For this review, take the finished solid that the model builds, in its own axes (mm). Round coordinates to 2 decimals unless told otherwise and drop trailing zeros. Write each loop counter-clockwise with the first axis right and the second up, starting at its lowest first coordinate (ties: lowest second). Pieces come first, ordered by that corner, then holes. Notation, with made-up numbers: (8, 59) -> (35, 59) arc R28 ccw to (35, 88) -> close; hole circle Ø1 at (-20, 27). An arc over 180 degrees is marked (long way). Answer as CSV lines item,"result". Start each with the question number.
Item 1: Take a section at B-B on z = 657.5. Give the boundary of the cut face in (x, y), then the cut area to 3 significant figures.
Item 2: Take a section at A-A on y = -20. Give the boundary of the cut face in (x, z), then the cut area to 3 significant figures.
Item 3: Wall thickness on probe 1 along X at (y, z) = (-5, 666); probe 2 along X at (y, z) = (-4, 436.5); probe 3 along Y at (x, z) = (17.5, 52.5): over which ranges is each line inside the solid? List them lowest first. Write a range as from..to.
Item 4: For pin 1 Ø10 at (x, y) = (13.5, -9.5) entering from -Z (3 decimals), flat-tipped, find the tip position at first contact; note if it passes through.
Item 5: Mouldability with a two-part tool opening along X and no side actions: class faces 1 (the flat face through (32.5, -15, 493)), 2 (the flat face through (16.1, -1.6, 0)), 3 (the flat face through (30.5, -16, 493)), 4 (the flat face through (1.5, -16, 493)) as +X half, -X half, draft (parallel to the pull), parting line (faces both ways), or undercut.
```python
from build123d import *

# Parameters (mm, degrees)
EXTRUDE_1_DEPTH = 1000


with BuildPart() as part:
    # 草图1 → 凸台-拉伸1 (new body)
    with BuildSketch(Plane.XY):
        with BuildLine():
            Line((10.5, -30), (0, -30))
            ThreePointArc((0, -30), (-0.353553391, -29.853553391), (-0.5, -29.5))
            Line((-0.5, -29.5), (-0.5, -0.5))
            ThreePointArc((-0.5, -0.5), (-0.353553391, -0.146446609), (0, 0))
            Line((0, 0), (32, 0))
            ThreePointArc((32, 0), (32.353553391, -0.146446609), (32.5, -0.5))
            Line((32.5, -0.5), (32.5, -29.5))
            ThreePointArc((32.5, -29.5), (32.353553391, -29.853553391), (32, -30))
            Line((32, -30), (21.5, -30))
            Line((21.5, -30), (21.5, -27))
            ThreePointArc((21.5, -27), (25.038664483, -28.385121551), (28.838528773, -28.426827781))
            ThreePointArc((28.838528773, -28.426827781), (30.029224893, -27.744667111), (30.5, -26.455686418))
            Line((30.5, -26.455686418), (30.5, -5))
            ThreePointArc((30.5, -5), (29.621320344, -2.878679656), (27.5, -2))
            Line((27.5, -2), (21.562207583, -2))
            Line((21.562207583, -2), (21.175427925, -2.706444665))
            ThreePointArc((21.175427925, -2.706444665), (21, -2.810397577), (20.824572075, -2.706444665))
            Line((20.824572075, -2.706444665), (20.437792417, -2))
            Line((20.437792417, -2), (11.562207583, -2))
            Line((11.562207583, -2), (11.175427925, -2.706444665))
            ThreePointArc((11.175427925, -2.706444665), (11, -2.810397577), (10.824572075, -2.706444665))
            Line((10.824572075, -2.706444665), (10.437792417, -2))
            Line((10.437792417, -2), (4.5, -2))
            ThreePointArc((4.5, -2), (2.378679656, -2.878679656), (1.5, -5))
            Line((1.5, -5), (1.5, -26.455686418))
            ThreePointArc((1.5, -26.455686418), (1.970775107, -27.744667111), (3.161471227, -28.426827781))
            ThreePointArc((3.161471227, -28.426827781), (6.961335517, -28.385121551), (10.5, -27))
            Line((10.5, -27), (10.5, -30))
        make_face()
    extrude(amount=EXTRUDE_1_DEPTH)


solid = part.part
```
Output values:
1,outline,"(-0.5, -29.5) arc R0.5 ccw to (0, -30) -> (10.5, -30) -> (10.5, -27) arc R10.55 cw to (3.16, -28.43) arc R2 cw to (1.5, -26.46) -> (1.5, -5) arc R3 cw to (4.5, -2) -> (10.44, -2) -> (10.82, -2.71) arc R0.2 ccw to (11.18, -2.71) -> (11.56, -2) -> (20.44, -2) -> (20.82, -2.71) arc R0.2 ccw to (21.18, -2.71) -> (21.56, -2) -> (27.5, -2) arc R3 cw to (30.5, -5) -> (30.5, -26.46) arc R2 cw to (28.84, -28.43) arc R10.55 cw to (21.5, -27) -> (21.5, -30) -> (32, -30) arc R0.5 ccw to (32.5, -29.5) -> (32.5, -0.5) arc R0.5 ccw to (32, 0) -> (0, 0) arc R0.5 ccw to (-0.5, -0.5) -> close"
1,area,"216 mm^2"
2,outline,"(-0.5, 0) -> (1.5, 0) -> (1.5, 1000) -> (-0.5, 1000) -> close; (30.5, 0) -> (32.5, 0) -> (32.5, 1000) -> (30.5, 1000) -> close"
2,area,"4,000 mm^2"
3,probe 1,"x = -0.5..1.5, 30.5..32.5"
3,probe 2,"x = -0.5..1.67, 30.33..32.5"
3,probe 3,"y = -2..0"
4,pin 1,"passes through"
5,face 1,"+X half"
5,face 2,"draft"
5,face 3,"undercut"
5,face 4,"undercut"
